from build123d import *

# Parameters (mm, degrees)
SKETCH1_W           = 53
SKETCH1_H           = 12.5
BOSS_EXTRUDE1_DEPTH = 1
BOSS_EXTRUDE2_DEPTH = 5
SKETCH3_R           = 1.5
CUT_EXTRUDE1_DEPTH  = 28.682349973
FILLET1_R           = 1
FILLET2_R           = 0.5
BOSS_EXTRUDE3_DEPTH = 3.5
FILLET3_R           = 0.5


with BuildPart() as part:
    # Sketch1 → Boss-Extrude1 (new body)
    with BuildSketch(Plane.XY):
        Rectangle(SKETCH1_W, SKETCH1_H)
    extrude(amount=BOSS_EXTRUDE1_DEPTH)

    # Sketch2 → Boss-Extrude2 (add)
    with BuildSketch(Plane.XY.offset(1)):
        with BuildLine():
            Line((19.227555087, 2.9), (17.977555087, -2.9))
            ThreePointArc((17.977555087, -2.9), (17.628219716, -3.467356005), (17, -3.689320024))
            Line((17, -3.689320024), (-17, -3.689320024))
            ThreePointArc((-17, -3.689320024), (-17.628219716, -3.467356005), (-17.977555087, -2.9))
            Line((-17.977555087, -2.9), (-19.227555087, 2.9))
            ThreePointArc((-19.227555087, 2.9), (-19.028035981, 3.738899692), (-18.25, 4.110679976))
            Line((-18.25, 4.110679976), (18.25, 4.110679976))
            ThreePointArc((18.25, 4.110679976), (19.028035981, 3.738899692), (19.227555087, 2.9))
        make_face()
    extrude(amount=BOSS_EXTRUDE2_DEPTH)

    # Sketch3 → Cut-Extrude1 (cut, through all)
    with BuildSketch(Plane.XY.offset(1)):
        with Locations((-23, 0)):
            Circle(SKETCH3_R)
        with Locations(Location((23, 0, 0), (0, 0, 180))):
            Circle(SKETCH3_R)
    extrude(amount=-CUT_EXTRUDE1_DEPTH, mode=Mode.SUBTRACT)

    # Fillet1
    fillet1_edges = [part.edges().sort_by_distance(p)[0] for p in [
        (17.628219716, -3.467356005, 1),
        (18.602555087, 0, 1),
        (19.028035981, 3.738899692, 1),
        (0, 4.110679976, 1),
        (-19.028035981, 3.738899692, 1),
        (-18.602555087, 0, 1),
        (-17.628219716, -3.467356005, 1),
        (0, -3.689320024, 1),
    ]]
    fillet(fillet1_edges, radius=FILLET1_R)

    # Fillet2
    fillet2_edges = [part.edges().sort_by_distance(p)[0] for p in [
        (17.628219716, -3.467356005, 6),
        (18.602555087, 0, 6),
        (19.028035981, 3.738899692, 6),
        (0, 4.110679976, 6),
        (-19.028035981, 3.738899692, 6),
        (-18.602555087, 0, 6),
        (-17.628219716, -3.467356005, 6),
        (0, -3.689320024, 6),
        (26.5, -6.25, 0.5),
        (-26.5, -6.25, 0.5),
        (-26.5, 6.25, 0.5),
        (26.5, 6.25, 0.5),
    ]]
    fillet(fillet2_edges, radius=FILLET2_R)

    # Sketch5 → Boss-Extrude3 (add)
    with BuildSketch(Plane(origin=(0, 0, 0), x_dir=(-1, 0, 0), z_dir=(0, 0, -1))):
        with BuildLine():
            Line((-19.488477495, 5.110679976), (19.488477495, 5.110679976))
            ThreePointArc((19.488477495, 5.110679976), (20.266513476, 4.738899692), (20.466032582, 3.9))
            Line((20.466032582, 3.9), (18.7849981, -3.9))
            ThreePointArc((18.7849981, -3.9), (18.435662729, -4.467356005), (17.807443013, -4.689320024))
            Line((17.807443013, -4.689320024), (-17.807443013, -4.689320024))
            ThreePointArc((-17.807443013, -4.689320024), (-18.435662729, -4.467356005), (-18.7849981, -3.9))
            Line((-18.7849981, -3.9), (-20.466032582, 3.9))
            ThreePointArc((-20.466032582, 3.9), (-20.266513476, 4.738899692), (-19.488477495, 5.110679976))
        make_face()
    extrude(amount=BOSS_EXTRUDE3_DEPTH)

    # Fillet3
    fillet3_edges = [part.edges().sort_by_distance(p)[0] for p in [
        (18.435662729, -4.467356005, 0),
        (0, -4.689320024, 0),
        (-18.435662729, -4.467356005, 0),
        (-19.625515341, 0, 0),
        (-20.266513476, 4.738899692, 0),
        (0, 5.110679976, 0),
        (20.266513476, 4.738899692, 0),
        (19.625515341, 0, 0),
        (18.435662729, -4.467356005, -3.5),
        (0, -4.689320024, -3.5),
        (-18.435662729, -4.467356005, -3.5),
        (-19.625515341, 0, -3.5),
        (-20.266513476, 4.738899692, -3.5),
        (0, 5.110679976, -3.5),
        (20.266513476, 4.738899692, -3.5),
        (19.625515341, 0, -3.5),
    ]]
    fillet(fillet3_edges, radius=FILLET3_R)


solid = part.part
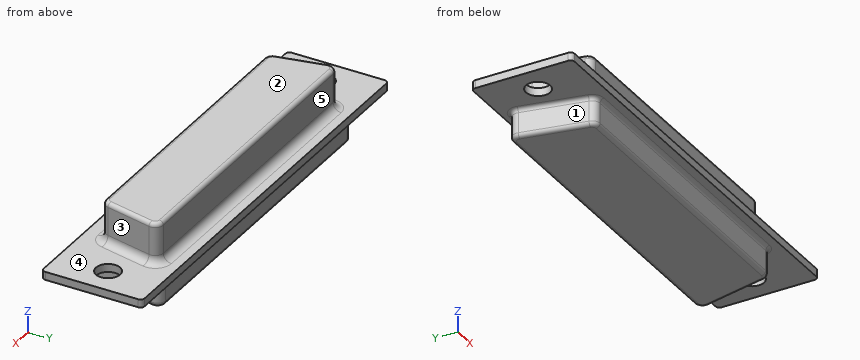
Build history of the part. All positions in model axes, mm. Face numbers are marked on the shaded views. A direction names the side the tool comes from. Round coordinates to 2 decimals unless told otherwise and drop trailing zeros. Write each loop counter-clockwise with the first axis right and the second up, starting at its lowest first coordinate (ties: lowest second). Pieces come first, ordered by that corner, then holes. Notation, with made-up numbers: (15, 48.25) -> (70, 48.25) arc R32 cw to (70, 75.25) -> close; hole circle Ø5 at (-20, 56). An arc over 180 degrees is marked (long way). Use one line per item in the form item = value.
Q1. Drop flat-ended pins along their axis: P1, Ø4, axis at x = 2.5, z = 4, coming from the +Y side; P2, Ø0.8, axis at x = 3.5, z = -2, coming from the +Y side; P3, Ø0.8, axis at x = -5, z = -1.5, coming from the -Y side. Give the stop position or say it passes through.
Conclusion:
P1 = 4.11
P2 = 5.11
P3 = -4.69
Q2. Band-saw the part on A-A, the plane x = -23. Write the cut outline in (y, z), then the cut area to 3 significant figures.
Conclusion:
outline = (-6.25, 0) -> (-1.5, 0) -> (-1.5, 1) -> (-6.25, 1) -> close; (1.5, 0) -> (6.25, 0) -> (6.25, 1) -> (1.5, 1) -> close
area = 9.50 mm²
Q3. Tool access for the marked faces 1, 2, 3, 4 and 5: list every direction of +Z, -Z, +X, -X, +Y, -Y with a clear straight run to the whole face (end or side of a thin tool).
Conclusion:
face_1 = -Z, -X, -Y
face_2 = +Z, +X, -X, +Y, -Y
face_3 = +Z, +X, -Y
face_4 = +Z
face_5 = +Z, +X, -X, +Y
Q4. Band-saw the part on C-C, the plane x = 14. Write the cut outline in (y, z), then the cut area to 3 significant figures.
Conclusion:
outline = (-6.25, 0) -> (-5.19, 0) arc R0.5 cw to (-4.69, -0.5) -> (-4.69, -3) arc R0.5 ccw to (-4.19, -3.5) -> (4.61, -3.5) arc R0.5 ccw to (5.11, -3) -> (5.11, -0.5) arc R0.5 cw to (5.61, 0) -> (6.25, 0) -> (6.25, 1) -> (5.11, 1) arc R1 cw to (4.11, 2) -> (4.11, 5.5) arc R0.5 ccw to (3.61, 6) -> (-3.19, 6) arc R0.5 ccw to (-3.69, 5.5) -> (-3.69, 2) arc R1 cw to (-4.69, 1) -> (-6.25, 1) -> close
area = 86.1 mm²
Q5. Band-saw the part on D-D, the plane y = 0. State how many separate pieces and enclosed holes the cut face has, then the cut area to 3 significant figures.
Conclusion:
separate_pieces = 3
enclosed_holes = 0
area = 371 mm²
Q6. Band-saw the part on B-B, the plane z = 4.5. Write the cut outline in (x, y).
Conclusion:
outline = (-19.23, 2.9) -> (-17.98, -2.9) arc R1 ccw to (-17, -3.69) -> (17, -3.69) arc R1 ccw to (17.98, -2.9) -> (19.23, 2.9) arc R1 ccw to (18.25, 4.11) -> (-18.25, 4.11) arc R1 ccw to start
Q7. Drill centre lines: L1, parallel to Y at x = -23, z = 0.55; L2, parallel to Y at x = 4, z = 4.25; L3, parallel to Z at x = 10.5, y = 5.75. Where is each one in solid material? Low to high.
Conclusion:
L1 = -6.25 to -1.5, 1.5 to 6.25
L2 = -3.69 to 4.11
L3 = 0 to 1
